Work out the finished part from the listing and answer in its coordinate system (mm). Round coordinates to 2 decimals unless told otherwise and drop trailing zeros. Order: outer loops, then holes, each group sorted by start corner. A loop starts at its lowest first (then second) coordinate and runs counter-clockwise, first axis right, second up. Notation, with made-up numbers: (-25.75, -30) - (-10.75, -30) arc R18 cw to (-10.75, -1) - close; hole circle Ø7 at (-16.75, 84.25). An arc over 180 degrees is marked (long way). Use CSV: the item, a comma, the result in double quotes.
Autodesk Inventor part; units mm, degrees
ref_plane "YZ Plane" through (0, 0, 0) normal (1, 0, 0) x (0, 1, 0)
ref_plane "XZ Plane" through (0, 0, 0) normal (0, 1, 0) x (-1, 0, 0)
ref_plane "XY Plane" through (0, 0, 0) normal (0, 0, 1) x (1, 0, 0)
sketch "Sketch1" plane through (0, 0, 0) normal (0, 1, 0) x (-1, 0, 0)
  line L0 (0, 0) -> (150, 0)
  line L1 (150, 0) -> (150, -170)
  line L2 (150, -170) -> (0, -170)
  line L3 (0, -170) -> (0, 0)
  dimension "d0" = 150
  dimension "d1" = 170
extrude "Extrusion1" add sketch "Sketch1" along normal blind 5
sketch "Sketch2" plane through (0, 5, 0) normal (0, 1, 0) x (1, 0, 0)
  circle A0 centre (-30, 30) radius 3.75
  point P0 (0, 0)
  dimension "d4" = 7.5
extrude "Extrusion2" cut sketch "Sketch2" against normal blind 5
pattern_linear "Rectangular Pattern1" count 6 spacing 20 along (0, 0, -1) of "Extrusion2"
sketch "Sketch3" plane through (0, 5, 0) normal (0, 1, 0) x (1, 0, 0)
  circle A0 centre (-58, 30) radius 3
  point P0 (0, 0)
  dimension "d10" = 6
extrude "Extrusion3" cut sketch "Sketch3" against normal blind 5
pattern_linear "Rectangular Pattern2" count 2 spacing 20 along (-1, 0, 0) count 4 spacing 30 along (0, 0, -1) of "Extrusion3"
sketch "Sketch4" plane through (-150, 0, -170) normal (-1, 0, 0) x (0, 0, 1)
  line L0 (170, 5) -> (0, 5)
  line L1 (170, 0) -> (0, 0)
  line L2 (0, 0) -> (0, 5)
  line L3 (0, 5) -> (170, 5)
  line L4 (170, 5) -> (170, 0)
extrude "Extrusion4" cut sketch "Sketch4" against normal blind 59.75
properties part number "Switchboard"
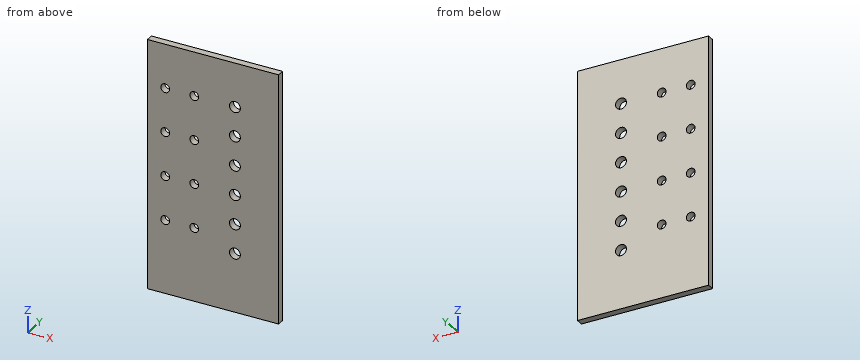
(1) Find section A-A (z = -130). Determine the outline of the cut face in (x, y).
Findings below:
outline,"(-90.25, 0) - (-33.75, 0) - (-33.75, 5) - (-90.25, 5) - close; (-26.25, 0) - (0, 0) - (0, 5) - (-26.25, 5) - close"
(2) Find section C-C (y = 0.95). State how many separate pieces and enclosed holes the cut face has, and give its area (3 significant figures).
Findings below:
separate pieces,"1"
enclosed holes,"14"
area,"14,900 mm²"
(3) Find section B-B (x = -30). Determine the outline of the cut face in (y, z), and give its area (3 significant figures).
Findings below:
outline,"(0, -170) - (5, -170) - (5, -133.75) - (0, -133.75) - close; (0, -126.25) - (5, -126.25) - (5, -113.75) - (0, -113.75) - close; (0, -106.25) - (5, -106.25) - (5, -93.75) - (0, -93.75) - close; (0, -86.25) - (5, -86.25) - (5, -73.75) - (0, -73.75) - close; (0, -66.25) - (5, -66.25) - (5, -53.75) - (0, -53.75) - close; (0, -46.25) - (5, -46.25) - (5, -33.75) - (0, -33.75) - close; (0, -26.25) - (5, -26.25) - (5, 0) - (0, 0) - close"
area,"625 mm²"
(4) Find section D-D (x = -58). Determine the outline of the cut face in (y, z), and give its area (3 significant figures).
Findings below:
outline,"(0, -170) - (5, -170) - (5, -123) - (0, -123) - close; (0, -117) - (5, -117) - (5, -93) - (0, -93) - close; (0, -87) - (5, -87) - (5, -63) - (0, -63) - close; (0, -57) - (5, -57) - (5, -33) - (0, -33) - close; (0, -27) - (5, -27) - (5, 0) - (0, 0) - close"
area,"730 mm²"
(5) This flat-tipped pin is pushed along its axis until it touches: pin 1 (7 mm diameter, centred on x = -30, z = -70, fed in from +Y). Where does it stop, or does it pass through?
Findings below:
pin 1,"passes through"
(6) Find the intervals of material crossed by L1, parallel to X at y = 3.95, z = -90; L2, parallel to X at y = 2.1, z = -60; L3, parallel to X at y = 2.95, z = -50, in increasing order. Write a range as from..to.
Findings below:
L1,"x = -90.25..-81, -75..-61, -55..-33.75, -26.25..0"
L2,"x = -90.25..-81, -75..-61, -55..0"
L3,"x = -90.25..-33.75, -26.25..0"
